Check sheet for the modelled part. Datum: model origin and axes. Units: mm. Face numbers are marked on the shaded views. A direction names the side the tool comes from. Give positions to 0.01 mm unless a question says otherwise; leave off trailing zeros. Order: outer loops, then holes, each group sorted by start corner. A loop starts at its lowest first (then second) coordinate and runs counter-clockwise, first axis right, second up. Notation, with made-up numbers: M 47.25,-35 L 64.25,-35 A26 cw 64.25,4 Z; hole C 42.25,69 d3. An arc over 180 degrees is marked long. Return JSON: item names as keys, results as strings. Group by question number.
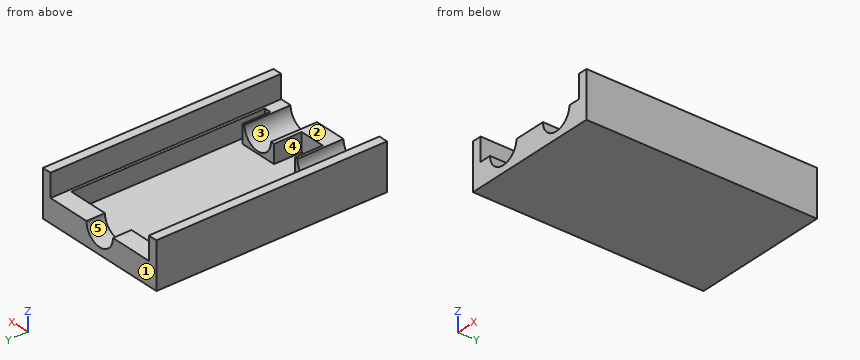
from build123d import *

# Parameters (mm, degrees)
PAD_DEPTH      = 25
SKETCH001_R    = 1.75
HOLE_DEPTH     = 5
HOLE_TIPS_R    = 1.75
POCKET_DEPTH   = 2
SKETCH003_R    = 1.75
HOLE001_DEPTH  = 2
HOLE001_TIPS_R = 1.75


with BuildPart() as part:
    # Sketch → Pad (new body)
    with BuildSketch(Plane.XZ):
        Polygon((0, 0), (15, 0), (15, 5), (14, 5), (14, 2.5), (1, 2.5), (1, 5), (0, 5), align=None)
    extrude(amount=PAD_DEPTH)

    # Sketch001 (on Face10 of Pad) → Hole (cut)
    with BuildSketch(Plane.XZ.offset(25)):
        with Locations((4, 2.5)):
            Circle(SKETCH001_R)
        with Locations((11, 2.5)):
            Circle(SKETCH001_R)
    extrude(amount=-HOLE_DEPTH, mode=Mode.SUBTRACT)

    # Hole tips → Hole tip 1 section 0
    with BuildSketch(Plane.XZ.offset(20), mode=Mode.PRIVATE) as hole_tip_1_s0:
        with Locations((4, 2.5)):
            Circle(HOLE_TIPS_R)
    loft([hole_tip_1_s0.sketch, Vertex(4, -18.948494, 2.5)], mode=Mode.SUBTRACT)

    # Hole tips → Hole tip 2 section 0
    with BuildSketch(Plane.XZ.offset(20), mode=Mode.PRIVATE) as hole_tip_2_s0:
        with Locations((11, 2.5)):
            Circle(HOLE_TIPS_R)
    loft([hole_tip_2_s0.sketch, Vertex(11, -18.948494, 2.5)], mode=Mode.SUBTRACT)

    # Sketch002 (on Face2 of Hole) → Pocket (cut)
    with BuildSketch(Plane(origin=(0, 0, 2.5), x_dir=(-1, 0, 0), z_dir=(0, 0, 1))):
        Polygon((-13.7, 23), (-13, 23), (-13, 20), (-8.84, 20), (-8.84, 23), (-6.04, 23), (-6.04, 20), (-2, 20), (-2, 23), (-1.3, 23), (-1.3, 2), (-13.7, 2), align=None)
    extrude(amount=-POCKET_DEPTH, mode=Mode.SUBTRACT)

    # Sketch003 (on Face4 of Pocket) → Hole001 (cut)
    with BuildSketch(Plane(origin=(0, 0, 0), x_dir=(1, 0, 0), z_dir=(0, 1, 0))):
        with Locations((7.5, -2.5)):
            Circle(SKETCH003_R)
    extrude(amount=-HOLE001_DEPTH, mode=Mode.SUBTRACT)

    # Hole001 tips → Hole001 tip 1 section 0
    with BuildSketch(Plane(origin=(0, -2, 0), x_dir=(1, 0, 0), z_dir=(0, 1, 0)), mode=Mode.PRIVATE) as hole001_tip_1_s0:
        with Locations((7.5, -2.5)):
            Circle(HOLE001_TIPS_R)
    loft([hole001_tip_1_s0.sketch, Vertex(7.5, -3.051506, 2.5)], mode=Mode.SUBTRACT)


solid = part.part
1) Sectioned sample at A-A on y = -10.25. Record the boundary of the cut face in (x, z), then the cut area to 3 significant figures.
2) Sectioned sample at B-B on x = 7.5. Record the boundary of the cut face in (y, z).
3) Depth check by flat-ended pin: P1, Ø1, axis at y = -14.5, z = 1, coming from the -X side; P2, Ø2, axis at x = 10.5, y = -12.5, coming from the +Z side; P3, Ø4, axis at x = 7.5, y = -23.5, coming from the +Z side. Enter the tip coordinate at first touch or a pass-through.
4) Sectioned sample at D-D on x = 11. Record the boundary of the cut face in (y, z), then the cut area to 4 significant figures.
5) Tool access check on the marked faces 1, 2, 3, 4 and 5. Record the directions out of +Z, -Z, +X, -X, +Y, -Y that give a thin tool (end or side, any length) a straight path to the whole face; none if there is none.
6) Sectioned sample at C-C on y = -20.75. Record the boundary of the cut face in (x, z).
7) Material ranges on line 1 along X through (y, z) = (-12, 2.85); line 2 along X through (y, z) = (-9, 0.9); line 3 along X through (y, z) = (-20.25, 1.5), recorded low to high.
Reply:
{
 "1": {"outline": "M 0,0 L 15,0 L 15,5 L 14,5 L 14,2.5 L 13.7,2.5 L 13.7,0.5 L 1.3,0.5 L 1.3,2.5 L 1,2.5 L 1,5 L 0,5 Z", "area": "17.7 mm^2"},
 "2": {"outline": "M -25,0 L 0,0 L 0,0.75 L -2,0.75 L -2,0.5 L -23,0.5 L -23,2.5 L -25,2.5 Z"},
 "3": {"P1": "x = 0", "P2": "z = 0.5", "P3": "z = 2.5"},
 "4": {"outline": "M -25,0 L 0,0 L 0,2.5 L -2,2.5 L -2,0.5 L -20,0.5 L -20,0.75 L -25,0.75 Z", "area": "17.75 mm^2"},
 "5": {"face 1": "+Z, -Z, +X, -X, +Y", "face 2": "+Z, +Y, -Y", "face 3": "+Z, -Y", "face 4": "+Z", "face 5": "+Z, +Y"},
 "6": {"outline": "M 0,0 L 15,0 L 15,5 L 14,5 L 14,2.5 L 13.7,2.5 L 13.7,0.5 L 13,0.5 L 13,2.5 L 12.75,2.5 A1.75 cw 9.25,2.5 L 8.84,2.5 L 8.84,0.5 L 6.04,0.5 L 6.04,2.5 L 5.75,2.5 A1.75 cw 2.25,2.5 L 2,2.5 L 2,0.5 L 1.3,0.5 L 1.3,2.5 L 1,2.5 L 1,5 L 0,5 Z"},
 "7": {"line 1": "0 to 1, 14 to 15", "line 2": "0 to 1.3, 13.7 to 15", "line 3": "0 to 1.3, 2 to 2.56, 5.44 to 6.04, 8.84 to 9.56, 12.44 to 13, 13.7 to 15"}
}
